from build123d import *

# Parameters (mm, degrees)
F1_DEPTH = 63.5
F2_DEPTH = 25.4
F3_DEPTH = 7.9375


with BuildPart() as f1:
    # F0 (on Front) → F1 (new body, symmetric)
    with BuildSketch(Plane.XZ):
        Polygon((26.376324, 9.525), (-41.275, 9.525), (-41.275, -9.525), (41.275, -9.525), (41.275, 9.525), align=None)
    extrude(amount=F1_DEPTH, both=True)

    # F0 (on Front) → F2 (join, symmetric)
    with BuildSketch(Plane.XZ):
        with BuildLine():
            Line((26.376324, 28.684646), (26.376324, 9.525))
            Line((26.376324, 9.525), (41.275, 9.525))
            Line((41.275, 9.525), (41.275, 28.684646))
            ThreePointArc((41.275, 28.684646), (45.538798, 39.510339), (56.039803, 44.520778))
            Line((56.039803, 44.520778), (56.039803, 59.43829))
            ThreePointArc((56.039803, 59.43829), (53.712029, 59.265678), (51.404034, 58.917129))
            ThreePointArc((51.404034, 58.917129), (33.44511, 48.308543), (26.376324, 28.684646))
        make_face()
        Polygon((56.039803, 66.675), (56.039803, 59.43829), (56.039803, 44.520778), (56.039803, 38.144724), (56.039803, 38.1), (106.839803, 38.1), (106.839803, 66.675), align=None)
    extrude(amount=F2_DEPTH, both=True)

    # F0 (on Front) → F3 (join, symmetric)
    with BuildSketch(Plane.XZ):
        with BuildLine():
            add(Edge.make_bspline(
                [(-41.275, 9.525), (-21.080984, 43.4733), (9.512173, 56.584653), (51.404034, 58.917129)],
                knots=[0, 0, 0, 0, 105.018978, 105.018978, 105.018978, 105.018978], degree=3))
            Line((-41.275, 9.525), (26.376324, 9.525))
            Line((26.376324, 9.525), (26.376324, 28.684646))
            ThreePointArc((26.376324, 28.684646), (33.44511, 48.308543), (51.404034, 58.917129))
        make_face()
    extrude(amount=F3_DEPTH, both=True)


solid = f1.part
Design review of the part built by this model. Coordinates are the model's own, in mm. A direction names the side the tool comes from. Coordinates: 2 decimals unless noted, no trailing zeros. Loops run counter-clockwise (first coordinate to the right, second up) from the corner with the lowest first, then second, coordinate; pieces in that order, holes last. Notation, with made-up numbers: (-2, 68) -> (3, 68) arc R21 cw to (3, 83) -> close; hole circle Ø2 at (78, 27). An arc over 180 degrees is marked (long way). Use a Markdown table: item, result. Add a question column.
Item 1: Clearance check with flat-ended pins moving along their axes: P1, Ø1, axis at x = 83, z = 41.5, coming from the -Y side; P2, Ø19, axis at y = -27, z = 6, coming from the +X side (3 decimals); P3, Ø24.5, axis at x = 7.5, z = 37, coming from the +Y side. State where each tip first meets the part, or that it passes through.
Item 2: We need section A-A, the plane y = 18.5. Write out the cut boundary in (x, z) (3 decimals).
Item 3: We need section C-C, the plane x = 82. Write out the cut boundary in (y, z) (3 decimals), and give its area (3 significant figures).
Item 4: We need section B-B, the plane z = 0. Write out the cut boundary in (x, y) (3 decimals).
Item 5: Machinability: for faces 1 (the cylindrical face through (33.64, -16.79, 48.54)), 2 (the flat face through (81, 0, 38.1)), 3 (the flat face through (66, -25.4, 45)), which of the approach directions +Z, -Z, +X, -X, +Y, -Y give a long, thin tool a straight path to every point of the face, cutting with its end or side? Answer none if there is none.
Item 6: The part is to be moulded in two halves that separate along X. For faces 4 (the cylindrical face through (45.43, -0.36, 39.39)), 5 (the flat face through (-1, -63.5, 0)), 6 (the flat face through (-41.275, -1, 0)), say which applies: +X half, -X half, draft (parallel to the pull), parting line (faces both ways), or undercut.
Item 7: Wall thickness on L1, parallel to Z at x = -14, y = 52 (3 decimals); L2, parallel to X at y = -21.5, z = 1.5 (3 decimals); L3, parallel to X at y = 14, z = 62: over which ranges is each line inside the solid? List them lowest first. Write a range as from..to.
Numbers:
| question | item | result |
|---|---|---|
| 1 | P1 | stops at y = -25.4 |
| 1 | P2 | stops at x = 41.275 |
| 1 | P3 | stops at y = 7.94 |
| 2 | outline | (-41.275, -9.525) -> (41.275, -9.525) -> (41.275, 28.685) arc R15.875 cw to (56.04, 44.521) -> (56.04, 38.1) -> (106.84, 38.1) -> (106.84, 66.675) -> (56.04, 66.675) -> (56.04, 59.438) arc R30.774 ccw to (51.404, 58.917) arc R30.774 ccw to (26.376, 28.685) -> (26.376, 9.525) -> (-41.275, 9.525) -> close |
| 3 | outline | (-25.4, 38.1) -> (25.4, 38.1) -> (25.4, 66.675) -> (-25.4, 66.675) -> close |
| 3 | area | 1,450 mm^2 |
| 4 | outline | (-41.275, -63.5) -> (41.275, -63.5) -> (41.275, 63.5) -> (-41.275, 63.5) -> close |
| 5 | face 1 | +Z, -X, -Y |
| 5 | face 2 | -Z, +X, +Y, -Y |
| 5 | face 3 | +Z, +X, -X, -Y |
| 6 | face 4 | undercut |
| 6 | face 5 | draft |
| 6 | face 6 | -X half |
| 7 | L1 | z = -9.525..9.525 |
| 7 | L2 | x = -41.275..41.275 |
| 7 | L3 | x = 56.04..106.84 |
